Read the model definition and answer for the solid it produces. Units are mm, in the model's axes. A direction names the side the tool comes from. Coordinates: 2 decimals unless noted, no trailing zeros. Loops run counter-clockwise (first coordinate to the right, second up) from the corner with the lowest first, then second, coordinate; pieces in that order, holes last. Notation, with made-up numbers: (83.5, 24.25) - (108.5, 24.25) arc R12 cw to (108.5, 31.25) - close; hole circle Ø1 at (69.5, -39.5). An arc over 180 degrees is marked (long way). Use one line per item in the form item = value. Start each with the question number.
1) Each of these flat-tipped pins is pushed along its axis until it touches: P1, Ø3, axis at x = -0.5, y = -1.5, coming from the +Z side; P2, Ø2.5, axis at x = 0, y = 0, coming from the -Z side. Where does it stop, or does it pass through?
2) The mould has two halves that part along Y. Classify faces 3 (the face through (1.146, -0.475, -0.129)), 4 (the face through (0, 0, -3.77)), 5 (the face through (0, 0, 0)): released by +Y, released by -Y, zero draft, split by the parting line, or undercut.
3) Which of the six approach directions +Z, -Z, +X, -X, +Y, -Y give full straight-line access (tool end or side, diameter ignored) to faces 1 (the face through (-0.5, -1.5, -5.556)), 2 (the face through (0.6, -1.03, -4.68))?
4) A cutting plane is placed at B-B (z = -3.3). Give the vertices of the cut face in (x, y), and give its area (3 significant figures).
5) A cutting plane is placed at A-A (z = -4.5). Give the vertices of the cut face in (x, y).
6) Consider line 1 (Z direction, x = -1.8, y = -0.9); line 2 (X direction, y = 0.15, z = -4.4); line 3 (X direction, y = -1.3, z = -4.8). Determine where each line is inside the solid, lowest interval first.
from build123d import *

# Parameters (mm, degrees)
SKETCH1_R          = 1.5875
EXTRUDE1_DEPTH     = 2.38125
CHAMFER3_SIZE      = 0.47625
CUT_SWEEP1_PITCH   = 0.635
SKETCH6_R          = 2.6035
EXTRUDE2_DEPTH     = 3.175
CUT_EXTRUDE1_DEPTH = 1.7859375
SKETCH8_R          = 1.374815329
CUT_EXTRUDE2_DEPTH = 0.3175
CUT_EXTRUDE2_DRAFT = -45
CHAMFER1_SIZE      = 0.3175
CHAMFER2_SIZE      = 0.15875


with BuildPart() as part:
    # Sketch1 → Extrude1 (new body)
    with BuildSketch(Plane.XY):
        Circle(SKETCH1_R)
    extrude(amount=-EXTRUDE1_DEPTH)

    # Chamfer3
    chamfer3_edges = [part.edges().sort_by_distance(p)[0] for p in [
        (-1.5875, 0, 0),
    ]]
    chamfer(chamfer3_edges, length=CHAMFER3_SIZE)

    # Cut-Sweep1: the profile of Sketch3 profile screwed along a right-hand helix of 4.75 turns, 6 arcs to a turn; built about Z, then put on its axis
    cut_sweep1_z = Axis((0, 0, 0), (0, 0, 1))
    cut_sweep1_corners = [(1.5878, 0, -0.555798205), (1.175055401, 0, -0.3175), (1.175055401, 0, -0.238125), (1.5878, 0, 0.000173205)]
    with BuildLine(mode=Mode.PRIVATE) as cut_sweep1_profile:
        Line(cut_sweep1_corners[0], cut_sweep1_corners[1])
        Line(cut_sweep1_corners[1], cut_sweep1_corners[2])
        Line(cut_sweep1_corners[2], cut_sweep1_corners[3])
        Line(cut_sweep1_corners[3], cut_sweep1_corners[0])
    cut_sweep1_cap = Face(cut_sweep1_profile.wire())
    cut_sweep1_turn_angles = [0, 30, 60, 90, 120, 150, 180, 210, 240, 270, 300, 330, 360]
    cut_sweep1_turn_weights = [1, 0.8660254037844387, 1, 0.8660254037844387, 1, 0.8660254037844387, 1, 0.8660254037844387, 1, 0.8660254037844387, 1, 0.8660254037844387, 1]
    cut_sweep1_turn_rails = [Edge.make_bspline([Vector(p[0], p[1], 0).rotate(cut_sweep1_z, cut_sweep1_turn_angles[k]) / cut_sweep1_turn_weights[k] + Vector(0, 0, p[2] + CUT_SWEEP1_PITCH * cut_sweep1_turn_angles[k] / 360) for k in range(13)], [0, 0, 0, 1, 1, 2, 2, 3, 3, 4, 4, 5, 5, 6, 6, 6], 2, cut_sweep1_turn_weights) for p in cut_sweep1_corners]
    cut_sweep1_turn_sides = [Face.make_surface_from_curves(cut_sweep1_turn_rails[p[0]], cut_sweep1_turn_rails[p[1]]) for p in [(0, 1), (1, 2), (2, 3), (3, 0)]]
    cut_sweep1_last_angles = [1440, 1470, 1500, 1530, 1560, 1590, 1620, 1650, 1680, 1695, 1710]
    cut_sweep1_last_weights = [1, 0.8660254037844387, 1, 0.8660254037844387, 1, 0.8660254037844387, 1, 0.8660254037844387, 1, 0.9659258262890595, 1]
    cut_sweep1_last_rails = [Edge.make_bspline([Vector(p[0], p[1], 0).rotate(cut_sweep1_z, cut_sweep1_last_angles[k]) / cut_sweep1_last_weights[k] + Vector(0, 0, p[2] + CUT_SWEEP1_PITCH * cut_sweep1_last_angles[k] / 360) for k in range(11)], [0, 0, 0, 1, 1, 2, 2, 3, 3, 4, 4, 5, 5, 5], 2, cut_sweep1_last_weights) for p in cut_sweep1_corners]
    cut_sweep1_last_sides = [Face.make_surface_from_curves(cut_sweep1_last_rails[p[0]], cut_sweep1_last_rails[p[1]]) for p in [(0, 1), (1, 2), (2, 3), (3, 0)]]
    cut_sweep1 = Plane(origin=(0, 0, 0), x_dir=(0, 1, 0), z_dir=(0, 0, -1)) * Solid(Shell([*[p.moved(Location((0, 0, CUT_SWEEP1_PITCH * i))) for i in range(4) for p in cut_sweep1_turn_sides], *cut_sweep1_last_sides, cut_sweep1_cap, cut_sweep1_cap.rotate(cut_sweep1_z, 1710).moved(Location((0, 0, CUT_SWEEP1_PITCH * 1710 / 360)))]))
    add(cut_sweep1, mode=Mode.SUBTRACT)

    # Sketch6 → Extrude2 (add)
    with BuildSketch(Plane(origin=(0, 0, -2.38125), x_dir=(-1, 0, 0), z_dir=(0, 0, -1))):
        Circle(SKETCH6_R)
    extrude(amount=EXTRUDE2_DEPTH)

    # Sketch7 → Cut-Extrude1 (cut)
    with BuildSketch(Plane(origin=(0, 0, -5.55625), x_dir=(-1, 0, 0), z_dir=(0, 0, -1))):
        Polygon((0, 1.374815329), (-1.190625, 0.687407664), (-1.190625, -0.687407664), (0, -1.374815329), (1.190625, -0.687407664), (1.190625, 0.687407664), align=None)
    extrude(amount=-CUT_EXTRUDE1_DEPTH, mode=Mode.SUBTRACT)


with BuildPart() as cut_extrude2_tool:
    # Sketch8 → Cut-Extrude2 (with draft: the straight prism first)
    with BuildSketch(Plane(origin=(0, 0, -5.55625), x_dir=(-1, 0, 0), z_dir=(0, 0, -1))):
        Circle(SKETCH8_R)
    extrude(amount=-CUT_EXTRUDE2_DEPTH)
    # Cut-Extrude2: the draft: its side faces are tilted about the plane it starts from
    cut_extrude2_sides = [cut_extrude2_tool.faces().sort_by_distance(p)[0] for p in [
        (1.374815329, 0, -5.3975),
    ]]
    draft(cut_extrude2_sides, Plane(origin=(0, 0, -5.55625), x_dir=(-1, 0, 0), z_dir=(0, 0, -1)), CUT_EXTRUDE2_DRAFT)


with BuildPart() as part_1:
    add(part.part)

    # Cut-Extrude2: cut by cut_extrude2_tool
    add(cut_extrude2_tool.part, mode=Mode.SUBTRACT)

    # Chamfer1
    chamfer1_edges = [part_1.edges().sort_by_distance(p)[0] for p in [
        (2.6035, 0, -5.55625),
    ]]
    chamfer(chamfer1_edges, length=CHAMFER1_SIZE)

    # Chamfer2
    chamfer2_edges = [part_1.edges().sort_by_distance(p)[0] for p in [
        (2.6035, 0, -2.38125),
    ]]
    chamfer(chamfer2_edges, length=CHAMFER2_SIZE)


solid = part_1.part
Found:
q1.P1 = 0
q1.P2 = -5.43
q2.face_3 = split by the parting line
q2.face_4 = undercut
q2.face_5 = zero draft
q3.face_1 = -Z, +X, -X, +Y, -Y
q3.face_2 = -Z
q4.outline = circle Ø5.21 at (0, 0)
q4.area = 21.3 mm^2
q5.outline = circle Ø5.21 at (0, 0); hole (-1.19, -0.69) - (0, -1.37) - (1.19, -0.69) - (1.19, 0.69) - (0, 1.37) - (-1.19, 0.69) - close
q6.line_1 = -5.56 to -2.38
q6.line_2 = -2.6 to -1.19, 1.19 to 2.6
q6.line_3 = -2.26 to -0.13, 0.13 to 2.26
